Source: CAD feature listing. Evaluate the final solid. Frame: model axes, mm. Give positions to 0.01 mm unless a question says otherwise; leave off trailing zeros. Loops run counter-clockwise (first coordinate to the right, second up) from the corner with the lowest first, then second, coordinate; pieces in that order, holes last. Notation, with made-up numbers: M 40,82 L 73,82 A28 cw 73,118 Z; hole C -16.75,-22.75 d2. An arc over 180 degrees is marked long. Put each result on its own line as item: value. Start each with the question number.
```python
from build123d import *

# Parameters (mm, degrees)
F0_W     = 95.25
F0_H     = 76.2
F1_DEPTH = 25.4
F4_DEPTH = 25.401
F2_R     = 2.161228
F2_R_2   = 2.1916
F5_DEPTH = 76.201


with BuildPart() as f1:
    # F0 (on Front) → F1 (new body)
    with BuildSketch(Plane.XZ):
        with Locations((-9.567424, 4.836748)):
            Rectangle(F0_W, F0_H)
    extrude(amount=F1_DEPTH)

    # F3 (on face) → F4 (cut, through all)
    with BuildSketch(Plane(origin=(0, 0, 0), x_dir=(-1, 0, 0), z_dir=(0, 1, 0))):
        with BuildLine():
            ThreePointArc((26.380295, 4.836748), (21.455919, 16.725243), (9.567424, 21.649619))
            Line((9.567424, 21.649619), (9.567424, 4.836748))
            Line((9.567424, 4.836748), (26.380295, 4.836748))
        make_face()
        with BuildLine():
            Line((9.567424, 4.836748), (9.567424, 21.649619))
            ThreePointArc((9.567424, 21.649619), (-2.321071, 16.725243), (-7.245446, 4.836748))
            Line((-7.245446, 4.836748), (9.567424, 4.836748))
        make_face()
        with BuildLine():
            Line((26.380295, 4.836748), (9.567424, 4.836748))
            Line((9.567424, 4.836748), (9.567424, -11.976122))
            ThreePointArc((9.567424, -11.976122), (21.455919, -7.051746), (26.380295, 4.836748))
        make_face()
        with BuildLine():
            Line((9.567424, -11.976122), (9.567424, 4.836748))
            Line((9.567424, 4.836748), (-7.245446, 4.836748))
            ThreePointArc((-7.245446, 4.836748), (-2.321071, -7.051746), (9.567424, -11.976122))
        make_face()
    extrude(amount=-F4_DEPTH, mode=Mode.SUBTRACT)

    # F2 (on face) → F5 (cut, through all)
    with BuildSketch(Plane.XY.offset(42.936748)):
        with Locations((28.788551, -12.7)):
            Circle(F2_R)
        with Locations((-47.411449, -12.7)):
            Circle(F2_R_2)
    extrude(amount=-F5_DEPTH, mode=Mode.SUBTRACT)


solid = f1.part
```
1. Section A-A, the plane y = -12.7. Output: boundary loops of the cut face in (x, z).
2. Ray query, line 1 (X direction, y = -12.5, z = 10.5); line 2 (X direction, y = -11, z = -20); line 3 (Z direction, x = -23.5, y = -12.75). Return the intervals inside material, ascending.
3. Section D-D, the plane y = -6. Output: boundary loops of the cut face in (x, z), plus the area to 3 significant figures.
4. Section B-B, the plane z = 10. Output: boundary loops of the cut face in (x, y), plus the area to 3 significant figures.
5. Section C-C, the plane x = -2.5. Output: boundary loops of the cut face in (y, z).
6. Pull-direction query (Y, two-part tool) for faces 1 (the face through (38.058, -13, 4)), 2 (the face through (-49.03, -11.22, 5.37)), 3 (the face through (-10, -25.4, 22)), 4 (the face through (29.786, -14.617, 5.37)); classes: released by +Y, released by -Y, zero draft, split by the parting line, or undercut.
Results found:
1. outline: M -57.19,-33.26 L -49.6,-33.26 L -49.6,42.94 L -57.19,42.94 Z; M -45.22,-33.26 L 26.63,-33.26 L 26.63,42.94 L -45.22,42.94 Z; M 30.95,-33.26 L 38.06,-33.26 L 38.06,42.94 L 30.95,42.94 Z; hole M -26.38,4.84 A16.81 ccw -9.57,-11.98 A16.81 ccw 7.25,4.84 A16.81 ccw -9.57,21.65 A16.81 ccw Z
2. line 1: -57.19 to -49.59, -45.23 to -25.4, 6.26 to 26.64, 30.94 to 38.06
2. line 2: -57.19 to -48.79, -46.03 to 27.45, 30.12 to 38.06
2. line 3: -33.26 to -4.57, 14.25 to 42.94
3. outline: M -57.19,-33.26 L 38.06,-33.26 L 38.06,42.94 L -57.19,42.94 Z; hole M -26.38,4.84 A16.81 ccw -9.57,-11.98 A16.81 ccw 7.25,4.84 A16.81 ccw -9.57,21.65 A16.81 ccw Z
3. area: 6,370 mm²
4. outline: M -57.19,-25.4 L -25.57,-25.4 L -25.57,0 L -57.19,0 Z; M 6.43,-25.4 L 38.06,-25.4 L 38.06,0 L 6.43,0 Z; hole C -47.41,-12.7 d4.38; hole C 28.79,-12.7 d4.32
4. area: 1,580 mm²
5. outline: M -25.4,-33.26 L 0,-33.26 L 0,-10.42 L -25.4,-10.42 Z; M -25.4,20.09 L 0,20.09 L 0,42.94 L -25.4,42.94 Z
6. face 1: zero draft
6. face 2: undercut
6. face 3: released by -Y
6. face 4: undercut
